Build history of the part. All positions in model axes, mm. Give positions to 0.01 mm unless a question says otherwise; leave off trailing zeros. Write each loop counter-clockwise with the first axis right and the second up, starting at its lowest first coordinate (ties: lowest second). Pieces come first, ordered by that corner, then holes.
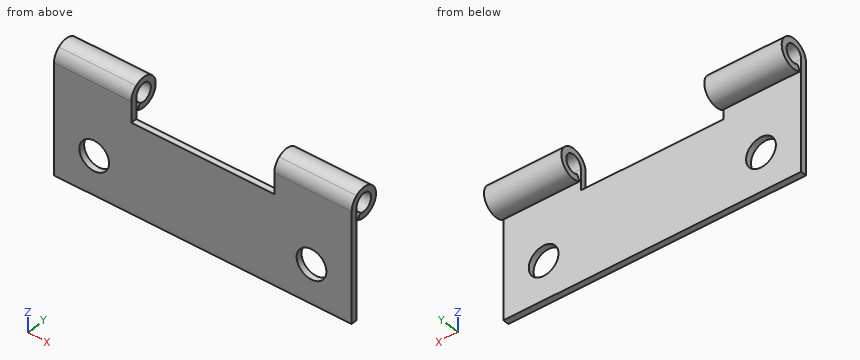
from build123d import *

# Parameters (mm, degrees)
SKETCH2_W               = 50
SKETCH2_H               = 21
BASE_FLANGE1_DEPTH      = 1
HEM1_START              = -25
HEM1_DEPTH              = 50
HEM1_2_DEPTH            = 50
CUT_EXTRUDE1_DEPTH      = 28.408940147
CUT_EXTRUDE1_DEPTH_BACK = 28.408940147
SKETCH5_W               = 24
SKETCH5_H               = 6
SKETCH6_R               = 2.5
CUT_EXTRUDE2_DEPTH      = 28.572631358


# Read off the part's stored shape, not the designer's step: Hem1
# Sheet-metal steps are written as plain solids
with BuildPart() as part:
    # Sketch2 → Base-Flange1 (new body)
    with BuildSketch(Plane(origin=(0, 0, 0), x_dir=(1, 0, 0), z_dir=(0, 1, 0))):
        Rectangle(SKETCH2_W, SKETCH2_H)
    extrude(amount=-BASE_FLANGE1_DEPTH)

    # Hem1 outline → Hem1 (cut)
    with BuildSketch(Plane.YZ.offset(HEM1_START)):
        with BuildLine():
            ThreePointArc((-1, 8), (-0.736067978, 9.118033989), (0, 10))
            Line((0, 10), (0, 10.5))
            Line((0, 10.5), (-1, 10.5))
            Line((-1, 10.5), (-1, 8))
        make_face()
    extrude(amount=HEM1_DEPTH, mode=Mode.SUBTRACT)

    # Hem1 2 outline → Hem1 2 (add)
    with BuildSketch(Plane.YZ.offset(HEM1_START)):
        with BuildLine():
            Line((0.75, 6.700961894), (0.25, 5.834936491))
            ThreePointArc((0.25, 5.834936491), (3.995508667, 8.149788152), (0, 10))
            Line((0, 10), (0, 8))
            ThreePointArc((0, 8), (2.799038106, 8.75), (0.75, 6.700961894))
        make_face()
    extrude(amount=HEM1_2_DEPTH)

    # Sketch5 → Cut-Extrude1 (cut, two sides: drawn at the far end of the back side and taken through both)
    with BuildSketch(Plane(origin=(0, 0, 0), x_dir=(1, 0, 0), z_dir=(0, 1, 0)).offset(-CUT_EXTRUDE1_DEPTH_BACK)):
        with Locations((0, -7.5)):
            Rectangle(SKETCH5_W, SKETCH5_H)
    extrude(amount=CUT_EXTRUDE1_DEPTH + CUT_EXTRUDE1_DEPTH_BACK, mode=Mode.SUBTRACT)

    # Sketch6 → Cut-Extrude2 (cut, through all)
    with BuildSketch(Plane.XZ.offset(1)):
        with Locations(Location((18.25, -4, 0), (0, 0, 270))):
            Circle(SKETCH6_R)
        with Locations(Location((-18.25, -4, 0), (0, 0, 270))):
            Circle(SKETCH6_R)
    extrude(amount=-CUT_EXTRUDE2_DEPTH, mode=Mode.SUBTRACT)


solid = part.part
(1) Probe line 1 (X direction, y = -0.4, z = -4); line 2 (X direction, y = -0.2, z = 6); line 3 (Z direction, x = -20.25, y = 1.5). List the from-to ranges inside material, lowest first.
(2) Saw through at D-D, the plane z = 1.25. List the corners of the cut face in (x, y).
(3) Drop flat-ended pins along their axis: pin 1 (6 mm diameter, centred on x = 18.25, z = -4, fed in from +Y); pin 2 (1.1 mm diameter, centred on x = 2, y = -0.5, fed in from +Z); pin 3 (4.5 mm diameter, centred on x = -18.25, z = -4, fed in from +Y). Give the stop position or say it passes through.
(4) Saw through at C-C, the plane x = -18.25. List the corners of the cut face in (y, z).
(5) Saw through at B-B, the plane y = 1.5. List the corners of the cut face in (x, z), plus the area to 3 significant figures.
(6) Saw through at A-A, the plane z = -4. List the corners of the cut face in (x, y), plus the area to 3 significant figures.
Computed values:
1. line 1: x = -25 to -20.75, -15.75 to 15.75, 20.75 to 25
1. line 2: x = -25 to -12, 12 to 25
1. line 3: z = 5.5 to 6.5, 9.5 to 10.5
2. outline: (-25, -1) - (25, -1) - (25, 0) - (-25, 0) - close
3. pin 1: stops at y = 0
3. pin 2: stops at z = 4.5
3. pin 3: passes through
4. outline: (-1, -10.5) - (0, -10.5) - (0, -6.5) - (-1, -6.5) - close; (-1, -1.5) - (0, -1.5) - (0, 8) arc R1.5 cw (long way) to (0.75, 6.7) - (0.25, 5.83) arc R2.5 ccw (long way) to (-1, 8) - close
5. outline: (-25, 5.5) - (-12, 5.5) - (-12, 6.5) - (-25, 6.5) - close; (-25, 9.5) - (-12, 9.5) - (-12, 10.5) - (-25, 10.5) - close; (12, 5.5) - (25, 5.5) - (25, 6.5) - (12, 6.5) - close; (12, 9.5) - (25, 9.5) - (25, 10.5) - (12, 10.5) - close
5. area: 52.0 mm2
6. outline: (-25, -1) - (-20.75, -1) - (-20.75, 0) - (-25, 0) - close; (-15.75, -1) - (15.75, -1) - (15.75, 0) - (-15.75, 0) - close; (20.75, -1) - (25, -1) - (25, 0) - (20.75, 0) - close
6. area: 40.0 mm2
